```python
from build123d import *

# Parameters (mm, degrees)
SKETCH1_W           = 70
SKETCH1_H           = 48
BOSS_EXTRUDE1_DEPTH = 1.5
BOSS_EXTRUDE2_DEPTH = 48
BOSS_EXTRUDE3_DEPTH = 1.5
BOSS_EXTRUDE4_DEPTH = 1.5
SKETCH9_R           = 5
BOSS_EXTRUDE5_DEPTH = 50
SKETCH10_R          = 2.8
CUT_EXTRUDE1_DEPTH  = 8
BOSS_EXTRUDE7_START = -50
BOSS_EXTRUDE7_DEPTH = 48.5
CUT_EXTRUDE4_DEPTH  = 52.511197813
CUT_EXTRUDE6_DEPTH  = 1.5


# Read off the part's stored shape, not the designer's step: Boss-Extrude7
with BuildPart() as part:
    # Sketch1 → Boss-Extrude1 (new body)
    with BuildSketch(Plane(origin=(0, 0, 0), x_dir=(1, 0, 0), z_dir=(0, 1, 0))):
        with Locations((-11.991596639, -2.521008403)):
            Rectangle(SKETCH1_W, SKETCH1_H)
    extrude(amount=BOSS_EXTRUDE1_DEPTH)

    # Sketch13 → Boss-Extrude2 (add)
    with BuildSketch(Plane.XY.offset(26.521008403)):
        Polygon((-46.991596639, 10), (-46.991596639, 1.5), (-45.491596639, 1.5), (-45.491596639, 9.010905763), (23.008403361, 38.36804862), (23.008403361, 40), align=None)
    extrude(amount=-BOSS_EXTRUDE2_DEPTH)

    # Sketch14 → Boss-Extrude3 (add)
    with BuildSketch(Plane.XY.offset(26.521008403)):
        Polygon((-46.991596639, 0), (23.008403361, 0), (23.008403361, 40), (-46.991596639, 10), align=None)
    extrude(amount=-BOSS_EXTRUDE3_DEPTH)

    # Sketch15 → Boss-Extrude4 (add)
    with BuildSketch(Plane(origin=(0, 0, -21.478991597), x_dir=(-1, 0, 0), z_dir=(0, 0, -1))):
        Polygon((-23.008403361, 0), (46.991596639, 0), (46.991596639, 10), (-23.008403361, 40), align=None)
    extrude(amount=-BOSS_EXTRUDE4_DEPTH)

    # Sketch9 → Boss-Extrude5 (add)
    with BuildSketch(Plane.XZ):
        with Locations(Location((-40.991596639, 2.521008403, 0), (0, 0, 270))):
            Circle(SKETCH9_R)
        with Locations(Location((-24.991596639, 20.521008403, 0), (0, 0, 270))):
            Circle(SKETCH9_R)
        with Locations(Location((17.008403361, 2.521008403, 0), (0, 0, 270))):
            Circle(SKETCH9_R)
        with Locations(Location((-24.991596639, -15.478991597, 0), (0, 0, 270))):
            Circle(SKETCH9_R)
    extrude(amount=-BOSS_EXTRUDE5_DEPTH)

    # Sketch10 → Cut-Extrude1 (cut)
    with BuildSketch(Plane.XZ):
        with Locations(Location((-40.991596639, 2.521008403, 0), (0, 0, 270))):
            Circle(SKETCH10_R)
        with Locations(Location((-24.991596639, 20.521008403, 0), (0, 0, 270))):
            Circle(SKETCH10_R)
        with Locations(Location((-24.991596639, -15.478991597, 0), (0, 0, 270))):
            Circle(SKETCH10_R)
        with Locations(Location((17.008403361, 2.521008403, 0), (0, 0, 270))):
            Circle(SKETCH10_R)
    extrude(amount=-CUT_EXTRUDE1_DEPTH, mode=Mode.SUBTRACT)

    # Boss-Extrude7 outline → Boss-Extrude7 (add)
    with BuildSketch(Plane.XZ.offset(BOSS_EXTRUDE7_START)):
        with BuildLine():
            ThreePointArc((-21.250723923, 17.203498596), (-21.79067464, 16.679902005), (-22.403055842, 16.243221996))
            Line((-22.403055842, 16.243221996), (-13.254543259, 5.265006896))
            ThreePointArc((-13.254543259, 5.265006896), (-9.913482791, 2.687784718), (-5.794711082, 1.771008403))
            Line((-5.794711082, 1.771008403), (12.064973378, 1.771008403))
            ThreePointArc((12.064973378, 1.771008403), (12.008403361, 2.521008403), (12.064973378, 3.271008403))
            Line((12.064973378, 3.271008403), (-5.092148663, 3.271008403))
            ThreePointArc((-5.092148663, 3.271008403), (-9.210920372, 4.187784718), (-12.55198084, 6.765006896))
            Line((-12.55198084, 6.765006896), (-21.250723923, 17.203498596))
        make_face()
    extrude(amount=BOSS_EXTRUDE7_DEPTH)

    # Sketch20 → Cut-Extrude4 (cut, through all)
    with BuildSketch(Plane(origin=(-10.912489134, 25.462474645, 0), x_dir=(0.9191450300180579, 0.3939192985791677, 0), z_dir=(-0.3939192985791677, 0.9191450300180579, 0))):
        with BuildLine():
            add(Edge.make_bspline(
                [(-15.317612613, 20.478991597), (-24.739688298, 20.478991597), (-20.028650455, 12.978991597), (-15.317612613, 5.478991597), (-10.606574771, 12.978991597), (-5.895536929, 20.478991597), (-15.317612613, 20.478991597)],
                knots=[4.71238898, 4.71238898, 4.71238898, 6.806784083, 6.806784083, 8.901179185, 8.901179185, 10.995574288, 10.995574288, 10.995574288], degree=2, weights=[1, 0.5, 1, 0.5, 1, 0.5, 1]))
        make_face()
        with BuildLine():
            add(Edge.make_bspline(
                [(24.998734434, -3.271008403), (26.776327601, -14.040210809), (34.50198737, -5.780609606), (42.227647139, 2.478991597), (30.377026022, 2.478991597)],
                knots=[0.150568273, 0.150568273, 0.150568273, 2.431478627, 2.431478627, 4.71238898, 4.71238898, 4.71238898], degree=2, weights=[1, 0.417180872, 1, 0.417180872, 1]))
            add(Edge.make_bspline(
                [(30.377026022, 2.478991597), (25.700250728, 2.478991597), (24.998734434, -1.771008403)],
                knots=[4.71238898, 4.71238898, 4.71238898, 6.132617034, 6.132617034, 6.132617034], degree=2, weights=[1, 0.758287544, 1]))
            Line((24.998734434, -1.771008403), (5.567976635, -1.771008403))
            add(Edge.make_bspline(
                [(5.567976635, -1.771008403), (0.619718616, -1.771008404), (-2.548078974, -5.265006896)],
                knots=[1.570796327, 1.570796327, 1.570796327, 2.446854377, 2.446854377, 2.446854377], degree=2, weights=[1, 0.905589421, 1]))
            Line((-2.548078974, -5.265006896), (-12.50136413, -16.243221996))
            add(Edge.make_bspline(
                [(-12.50136413, -16.243221996), (-13.799875321, -15.521008403), (-15.317612613, -15.521008403)],
                knots=[4.168218977, 4.168218977, 4.168218977, 4.71238898, 4.71238898, 4.71238898], degree=2, weights=[1, 0.963212666, 1]))
            add(Edge.make_bspline(
                [(-15.317612613, -15.521008403), (-22.262261076, -15.521008403), (-20.599158718, -21.718406923), (-18.936056359, -27.915805443), (-12.787966418, -24.947503117), (-6.639876476, -21.979200791), (-11.247664353, -17.203498596)],
                knots=[4.71238898, 4.71238898, 4.71238898, 6.525015233, 6.525015233, 8.337641486, 8.337641486, 10.150267739, 10.150267739, 10.150267739], degree=2, weights=[1, 0.616652372, 1, 0.616652372, 1, 0.616652372, 1]))
            Line((-11.247664353, -17.203498596), (-1.783713835, -6.765006896))
            add(Edge.make_bspline(
                [(6.332341775, -3.271008403), (1.384083756, -3.271008404), (-1.783713835, -6.765006896)],
                knots=[1.570796327, 1.570796327, 1.570796327, 2.446854377, 2.446854377, 2.446854377], degree=2, weights=[1, 0.905589421, 1]))
            Line((6.332341775, -3.271008403), (24.998734434, -3.271008403))
        make_face()
        with BuildLine():
            add(Edge.make_bspline(
                [(-32.725093998, 2.478991597), (-42.147169682, 2.478991597), (-37.43613184, -5.021008403), (-32.725093998, -12.521008403), (-28.014056156, -5.021008403), (-23.303018313, 2.478991597), (-32.725093998, 2.478991597)],
                knots=[4.71238898, 4.71238898, 4.71238898, 6.806784083, 6.806784083, 8.901179185, 8.901179185, 10.995574288, 10.995574288, 10.995574288], degree=2, weights=[1, 0.5, 1, 0.5, 1, 0.5, 1]))
        make_face()
    extrude(amount=CUT_EXTRUDE4_DEPTH, mode=Mode.SUBTRACT)


with BuildPart() as cut_extrude4_kept_piece:
    # of the separate pieces the step leaves, the one the design keeps (cut_extrude4_pieces_kept)
    add(part.part.solids().sort_by_distance((-46.991596639, 0, -21.478991597))[0])

    # Sketch22 → Cut-Extrude6 (cut)
    with BuildSketch(Plane.XZ):
        with BuildLine():
            Line((12.064973378, 3.271008403), (12.064973378, 25.021008403))
            Line((12.064973378, 25.021008403), (-22.812147167, 25.021008403))
            ThreePointArc((-22.812147167, 25.021008403), (-20.088442695, 21.500335417), (-21.250723923, 17.203498596))
            Line((-21.250723923, 17.203498596), (-12.55198084, 6.765006896))
            ThreePointArc((-12.55198084, 6.765006896), (-9.210920372, 4.187784718), (-5.092148663, 3.271008403))
            Line((-5.092148663, 3.271008403), (12.064973378, 3.271008403))
        make_face()
        with BuildLine():
            Line((-16.991596639, -19.978991597), (12.064973378, -19.978991597))
            Line((12.064973378, -19.978991597), (12.064973378, 1.771008403))
            Line((12.064973378, 1.771008403), (-5.794711082, 1.771008403))
            ThreePointArc((-5.794711082, 1.771008403), (-9.913482791, 2.687784718), (-13.254543259, 5.265006896))
            Line((-13.254543259, 5.265006896), (-22.403055842, 16.243221996))
            ThreePointArc((-22.403055842, 16.243221996), (-29.385253712, 18.134425591), (-27.17104611, 25.021008403))
            Line((-27.17104611, 25.021008403), (-32.991596639, 25.021008403))
            ThreePointArc((-32.991596639, 25.021008403), (-34.405810201, 24.435221966), (-34.991596639, 23.021008403))
            Line((-34.991596639, 23.021008403), (-34.991596639, -7.478991597))
            ThreePointArc((-34.991596639, -7.478991597), (-34.405810201, -8.893205159), (-32.991596639, -9.478991597))
            Line((-32.991596639, -9.478991597), (-20.991596639, -9.478991597))
            ThreePointArc((-20.991596639, -9.478991597), (-19.577383076, -10.064778034), (-18.991596639, -11.478991597))
            Line((-18.991596639, -11.478991597), (-18.991596639, -17.978991597))
            ThreePointArc((-18.991596639, -17.978991597), (-18.405810201, -19.393205159), (-16.991596639, -19.978991597))
        make_face()
    extrude(amount=-CUT_EXTRUDE6_DEPTH, mode=Mode.SUBTRACT)


solid = cut_extrude4_kept_piece.part
```
The listing builds one solid part. Answer for the finished solid, in the listing's coordinates (mm). A direction names the side the tool comes from. Round coordinates to 2 decimals unless told otherwise and drop trailing zeros. Loops run counter-clockwise (first coordinate to the right, second up) from the corner with the lowest first, then second, coordinate; pieces in that order, holes last.
Q1. Section D-D, the plane y = 30.5 is taken. Determine the outline of the cut face in (x, z).
Q2. Which of the six approach directions +Z, -Z, +X, -X, +Y, -Y give full straight-line access (tool end or side, diameter ignored) to faces 4 (the face through (-42.7, 3.94, 4.74)), 5 (the face through (-22.02, 10.59, -11.46)), 6 (the face through (-46.992, 5, 3))?
Q3. Section B-B, the plane z = 12.5 is taken. Determine the outline of the cut face in (x, y), then the cut area to 3 significant figures.
Q4. Given pin 1 Ø23 at (x, z) = (-33, -1) entering from +Y; pin 2 Ø12 at (y, z) = (24.5, 5) entering from -X; pin 3 Ø6.5 at (x, z) = (-24.99, -15.48) entering from +Y, each flat-ended and moving along its own axis, determine where each tip first touches the part or whether it passes through.
Q5. For a pull along Y with two mould halves and no side action, classify faces 1 (the face through (0, 15, -19.979)), 2 (the face through (-41, 8, 3)), 3 (the face through (-18.4, 0.7, -19.4)) as released by +Y, released by -Y, zero draft, split by the parting line, or undercut.
Q6. Find the intervals of material crossed by line 1 (X direction, y = 6, z = -13); line 2 (Z direction, x = -11.5, y = 17); line 3 (Z direction, x = 14.5, y = 32), in increasing order.
Q7. Section A-A, the plane z = -15.5 is taken. Determine the outline of the cut face in (x, y).
Q8. Section C-C, the plane x = -29 is taken. Determine the outline of the cut face in (y, z), then the cut area to 3 significant figures.
Completed:
1. outline: (0.84, -21.48) - (23.01, -21.48) - (23.01, -19.98) - (4.65, -19.98) - (4.65, 1.77) - (12.06, 1.77) arc R5 ccw (long way) to (12.06, 3.27) - (4.65, 3.27) - (4.65, 25.02) - (23.01, 25.02) - (23.01, 26.52) - (0.84, 26.52) - close
2. face 4: -Y
2. face 5: none
2. face 6: +Z, -Z, -X, +Y, -Y
3. outline: (-46.99, 0) - (-34.99, 0) - (-34.99, 1.5) - (-45.49, 1.5) - (-45.49, 9.01) - (-19.28, 20.24) - (-19.28, 0) - (-17.33, 0) - (-17.33, 21.08) - (23.01, 38.37) - (23.01, 40) - (-46.99, 10) - close; (12.06, 0) - (23.01, 0) - (23.01, 1.5) - (12.06, 1.5) - close
3. area: 200 mm2
4. pin 1: stops at y = 20.92
4. pin 2: stops at x = -27.16
4. pin 3: stops at y = 20.82
5. face 1: undercut
5. face 2: released by -Y
5. face 3: zero draft
6. line 1: x = -46.99 to -45.49, -29.33 to -26.29, -23.69 to -20.65
6. line 2: z = -21.48 to -19.98, 3.62 to 5.69, 25.02 to 26.52
6. line 3: z = -21.48 to -19.98, -1.8 to 6.85, 25.02 to 26.52
7. outline: (-46.99, 0) - (-27.79, 0) - (-27.79, 8) - (-22.19, 8) - (-22.19, 0) - (-18.99, 0) - (-18.99, 1.5) - (-19.99, 1.5) - (-19.99, 19.94) - (23.01, 38.37) - (23.01, 40) - (-46.99, 10) - close; (12.06, 0) - (23.01, 0) - (23.01, 1.5) - (12.06, 1.5) - close; hole (-45.49, 1.5) - (-29.99, 1.5) - (-29.99, 15.65) - (-45.49, 9.01) - close
8. outline: (0, -21.48) - (17.71, -21.48) - (17.71, 26.52) - (0, 26.52) - (0, 25.02) - (16.08, 25.02) - (16.08, 23.51) - (0, 23.51) - (0, 17.53) - (16.08, 17.53) - (16.08, -12.49) - (1.5, -12.49) - (1.5, -9.48) - (0, -9.48) - close; hole (1.5, -19.98) - (16.08, -19.98) - (16.08, -18.47) - (1.5, -18.47) - close
8. area: 326 mm2
